from build123d import *

# Parameters (mm, degrees)
F0_W     = 5
F0_H     = 5
F1_DEPTH = 3
F2_R     = 0.5
F3_DEPTH = 8
F4_R     = 0.5


with BuildPart() as f1:
    # F0 (on Top) → F1 (new body)
    with BuildSketch(Plane.XY):
        Rectangle(F0_W, F0_H)
    extrude(amount=F1_DEPTH)

    # F2 (on face) → F3 (join)
    with BuildSketch(Plane(origin=(0, 0, 0), x_dir=(1, 0, 0), z_dir=(0, 0, -1))):
        Circle(F2_R)
    extrude(amount=F3_DEPTH)

    # F4
    f4_edges = [f1.edges().sort_by_distance(p)[0] for p in [
        (-0.5, 0, -8),
    ]]
    fillet(f4_edges, radius=F4_R)


solid = f1.part
Could you check a few things on this model? Use its own coordinates, in mm. Coordinates: 2 decimals unless noted, no trailing zeros. Write each loop counter-clockwise with the first axis right and the second up, starting at its lowest first coordinate (ties: lowest second). Pieces come first, ordered by that corner, then holes. Notation, with made-up numbers: (51.25, 23) - (88.25, 23) arc R17 ccw to (88.25, 42) - close; hole circle Ø10 at (33.5, 23.25). An arc over 180 degrees is marked (long way). Put each result on its own line as item: value. Start each with the question number.
Q1. Please list where these lines run through material, in increasing order: L1, parallel to Z at x = -0.2, y = 2; L2, parallel to X at y = 0.25, z = -4.5; L3, parallel to Y at x = 0.2, z = -6.
Q2. I want a section at A-A on y = 0. Write out the boundary of the cut face in (x, z), plus the area to 3 significant figures.
Q3. Thinking about a two-plate mould opening in Y: for faces 1 (the cylindrical face through (-0.108, 0.488, -3.698)), 2 (the flat face through (2.5, 0, 1)), 3 (the flat face through (0, 2.5, 1)), 4 (the flat face through (0, -2.5, 1)), which applies, pulls with the +Y half, pulls with the -Y half, needs draft (parallel to the pull), parting line crosses it, or undercut?
Q4. I want a section at D-D on y = 1.8. Write out the boundary of the cut face in (x, z), plus the area to 3 significant figures.
Q5. I want a section at C-C on z = -6.5. Write out the boundary of the cut face in (x, y), plus the area to 3 significant figures.
Q6. I'm going to push flat-ended pins straight in: P1, Ø2, axis at y = -0.5, z = -2, coming from the +X side; P2, Ø1, axis at x = 0, z = -5, coming from the +Y side. Where does each tip first touch, or does it pass through?
Checks:
1. L1: 0 to 3
1. L2: -0.43 to 0.43
1. L3: -0.46 to 0.46
2. outline: (-2.5, 0) - (-0.5, 0) - (-0.5, -7.5) arc R0.5 ccw to (0.5, -7.5) - (0.5, 0) - (2.5, 0) - (2.5, 3) - (-2.5, 3) - close
2. area: 22.9 mm²
3. face 1: parting line crosses it
3. face 2: needs draft
3. face 3: pulls with the +Y half
3. face 4: pulls with the -Y half
4. outline: (-2.5, 0) - (2.5, 0) - (2.5, 3) - (-2.5, 3) - close
4. area: 15.0 mm²
5. outline: circle Ø1 at (0, 0)
5. area: 0.785 mm²
6. P1: x = 0.5
6. P2: y = 0.5
